Print and shaded views of the part. All mm, measured from the part's lowest x, y and z. Give positions to 0.01 mm unless a question says otherwise; leave off trailing zeros. Loops run counter-clockwise (first coordinate to the right, second up) from the corner with the lowest first, then second, coordinate; pieces in that order, holes last. Notation, with made-up numbers: M 5.25,-12.75 L 64.25,-12.75 A14 cw 64.25,-0.75 Z; hole C 60.25,15.25 d5. An arc over 180 degrees is marked long. Answer in a Markdown table with one row per item.
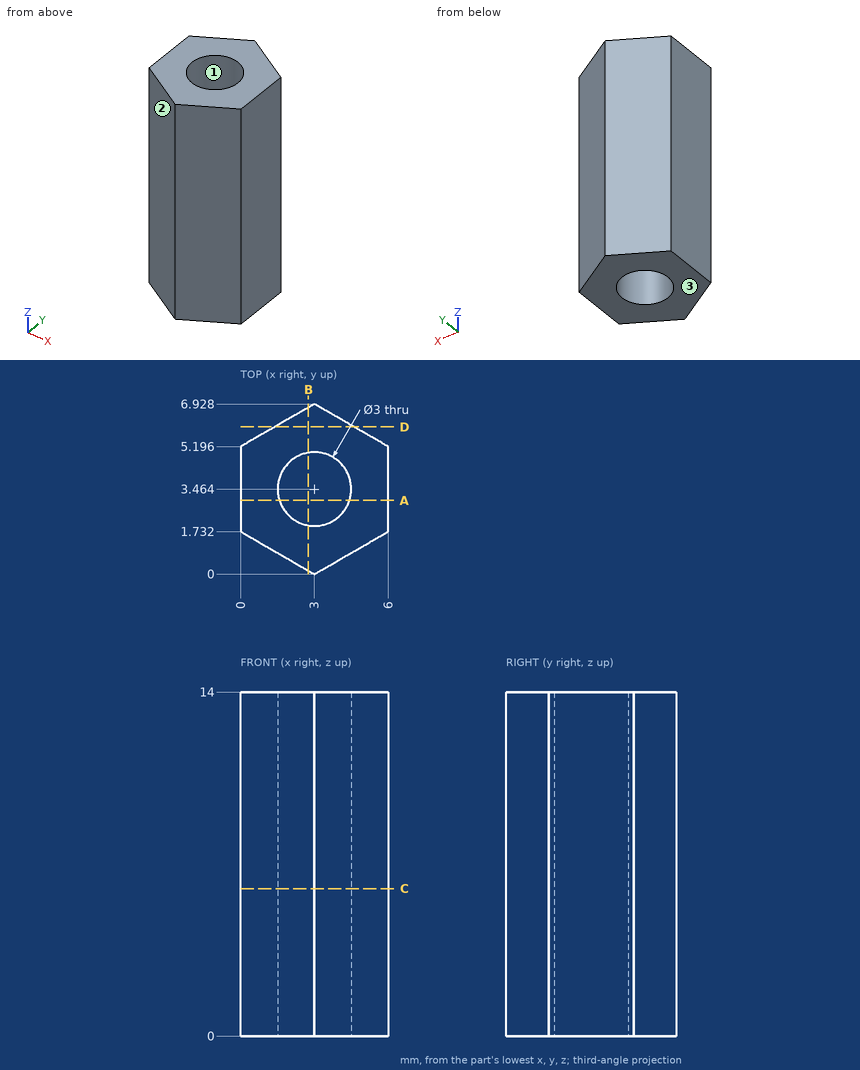
(1) Saw through at D-D, the plane y = 6. Give the cut face in (x, z), and give its area (3 significant figures).
Established:
| item | result |
|---|---|
| outline | M 1.39,0 L 4.61,0 L 4.61,14 L 1.39,14 Z |
| area | 45.0 mm2 |
(2) Saw through at A-A, the plane y = 3. Give the cut face in (x, z).
Established:
| item | result |
|---|---|
| outline | M 0,0 L 1.57,0 L 1.57,14 L 0,14 Z; M 4.43,0 L 6,0 L 6,14 L 4.43,14 Z |
(3) Saw through at C-C, the plane z = 6. Give the cut face in (x, y).
Established:
| item | result |
|---|---|
| outline | M 0,1.73 L 3,0 L 6,1.73 L 6,5.2 L 3,6.93 L 0,5.2 Z; hole C 3,3.46 d3 |
(4) Wall check: L1, parallel to X at y = 4.5, z = 3.5 (1 decimal); L2, parallel to X at y = 3.75, z = 12.25; L3, parallel to Y at x = 2.75, z = 1 (1 decimal). Give the ranges that are in metal, low to high.
Established:
| item | result |
|---|---|
| L1 | x = 0 to 1.9, 4.1 to 6 |
| L2 | x = 0 to 1.53, 4.47 to 6 |
| L3 | y = 0.1 to 2, 4.9 to 6.8 |
(5) Saw through at B-B, the plane x = 2.75. Give the cut face in (y, z) (1 decimal).
Established:
| item | result |
|---|---|
| outline | M 0.1,0 L 2,0 L 2,14 L 0.1,14 Z; M 4.9,0 L 6.8,0 L 6.8,14 L 4.9,14 Z |
(6) Mould opens along Y. For the marked faces 1, 2 and 3 say: pulls with the +Y half, pulls with the -Y half, needs draft (parallel to the pull), parting line crosses it, or undercut.
Established:
| item | result |
|---|---|
| face 1 | undercut |
| face 2 | pulls with the -Y half |
| face 3 | needs draft |
(7) Flat gauge pins, fed straight in: P1, Ø1.8, axis at x = 3, y = 3.46, coming from the -Z side; P2, Ø3, axis at x = 2, z = 5, coming from the +Y side. Where does each tip first touch, or does it go through?
Established:
| item | result |
|---|---|
| P1 | passes through |
| P2 | stops at y = 6.93 |
